```python
from build123d import *

# Parameters (mm, degrees)
SKETCH058_R     = 1.75
PAD036_DEPTH    = 5
SKETCH059_R     = 1.75
PAD037_DEPTH    = 0.6
SKETCH060_R     = 3
POCKET018_DEPTH = 3
SKETCH064_W     = 25
SKETCH064_H     = 15
POCKET020_DEPTH = 5
SKETCH065_W     = 32
SKETCH065_H     = 32
SKETCH065_W_2   = 25
SKETCH065_H_2   = 15
PAD040_DEPTH    = 3
POCKET021_DEPTH = 2
SKETCH067_W     = 32
SKETCH067_H     = 1.8
PAD041_DEPTH    = 2
SKETCH069_W     = 7.6
SKETCH069_H     = 1.2
PAD042_DEPTH    = 5
SKETCH070_R     = 1
POCKET022_DEPTH = 0.601
PAD043_DEPTH    = 10


with BuildPart() as part:
    # Sketch058 → Pad036 (new body)
    with BuildSketch(Plane.XY):
        Polygon((-42, 37.5), (12, 37.5), (12, 25.7), (42, 25.7), (42, -37.5), (-42, -37.5), align=None)
        with Locations((-15, 31.5)):
            Circle(SKETCH058_R, mode=Mode.SUBTRACT)
        with BuildLine():
            ThreePointArc((-18.5, 31.5), (-15, 28), (-11.5, 31.5))
            Line((-11.5, 31.5), (-11.5, 36.3))
            Line((-11.5, 36.3), (10.8, 36.3))
            Line((10.8, 36.3), (10.8, 24.5))
            Line((10.8, 24.5), (40.8, 24.5))
            Line((40.8, 24.5), (40.8, -36.3))
            Line((40.8, -36.3), (-40.8, -36.3))
            Line((-40.8, -36.3), (-40.8, 36.3))
            Line((-40.8, 36.3), (-18.5, 36.3))
            Line((-18.5, 31.5), (-18.5, 36.3))
        make_face(mode=Mode.SUBTRACT)
    extrude(amount=PAD036_DEPTH)

    # Sketch059 (on Face19 of Pad036) → Pad037 (join)
    with BuildSketch(Plane.XY.offset(5)):
        Polygon((-42, 37.5), (12, 37.5), (12, 25.7), (42, 25.7), (42, -37.5), (-42, -37.5), align=None)
        with Locations((-15, 31.5)):
            Circle(SKETCH059_R, mode=Mode.SUBTRACT)
    extrude(amount=PAD037_DEPTH)

    # Sketch060 (on Face1 of Pad037) → Pocket018 (cut)
    with BuildSketch(Plane.XY.offset(5.6)):
        with Locations((-15, 31.5)):
            Circle(SKETCH060_R)
    extrude(amount=-POCKET018_DEPTH, mode=Mode.SUBTRACT)

    # Sketch064 → Pocket020 (cut)
    with BuildSketch(Plane(origin=(0, 0, 5), x_dir=(1, 0, 0), z_dir=(0, 0, -1))):
        with Locations((-12.5, -7.5)):
            Rectangle(SKETCH064_W, SKETCH064_H)
    extrude(amount=-POCKET020_DEPTH, mode=Mode.SUBTRACT)

    # Sketch065 (on Face14 of Pocket020) → Pad040 (join)
    with BuildSketch(Plane(origin=(0, 0, 5), x_dir=(1, 0, 0), z_dir=(0, 0, -1))):
        with Locations((-12.5, -5)):
            Rectangle(SKETCH065_W, SKETCH065_H)
        with Locations((-12.5, -7.5)):
            Rectangle(SKETCH065_W_2, SKETCH065_H_2, mode=Mode.SUBTRACT)
    extrude(amount=PAD040_DEPTH)

    # Sketch066 (on Face24 of Pad040) → Pocket021 (cut)
    with BuildSketch(Plane(origin=(0, 0, 2), x_dir=(1, 0, 0), z_dir=(0, 0, -1))):
        Polygon((-26.75, -15.5), (-26.75, 5.5), (-21.75, 5.5), (-21.75, 9), (-3.25, 9), (-3.25, 5.5), (1.75, 5.5), (1.75, -15.5), (-3.25, -15.5), (-3.25, -19), (-21.75, -19), (-21.75, -15.5), align=None)
    extrude(amount=-POCKET021_DEPTH, mode=Mode.SUBTRACT)

    # Sketch067 (on Face40 of Pocket021) → Pad041 (join)
    with BuildSketch(Plane(origin=(0, 0, 2), x_dir=(1, 0, 0), z_dir=(0, 0, -1))):
        with Locations((-12.5, 10.1)):
            Rectangle(SKETCH067_W, SKETCH067_H)
        with Locations((-12.5, -20.1)):
            Rectangle(SKETCH067_W, SKETCH067_H)
    extrude(amount=PAD041_DEPTH)

    # Sketch069 (on Face13 of Pad041) → Pad042 (join)
    with BuildSketch(Plane(origin=(0, 0, 0), x_dir=(1, 0, 0), z_dir=(0, 0, -1))):
        with Locations((20.82, -25.1)):
            Rectangle(SKETCH069_W, SKETCH069_H)
    extrude(amount=PAD042_DEPTH)

    # Sketch070 (on Face40 of Pad042) → Pocket022 (cut, through all)
    with BuildSketch(Plane(origin=(0, 0, 5), x_dir=(1, 0, 0), z_dir=(0, 0, -1))):
        with Locations((24.892975, 0)):
            Circle(SKETCH070_R)
        with Locations((24.892975, -6)):
            Circle(SKETCH070_R)
        with Locations((24.892975, 6)):
            Circle(SKETCH070_R)
        with Locations((24.892975, 12)):
            Circle(SKETCH070_R)
    extrude(amount=-POCKET022_DEPTH, mode=Mode.SUBTRACT)

    # Sketch071 (on Face22 of Pocket022) → Pad043 (join)
    with BuildSketch(Plane(origin=(0, 0, 5), x_dir=(1, 0, 0), z_dir=(0, 0, -1))):
        with BuildLine():
            ThreePointArc((10.8, -32.3), (7.971573, -33.471573), (6.8, -36.3))
            Line((6.8, -36.3), (10.8, -36.3))
            Line((10.8, -36.3), (10.8, -32.3))
        make_face()
        with BuildLine():
            ThreePointArc((40.8, -20.5), (37.971573, -21.671573), (36.8, -24.5))
            Line((40.8, -24.5), (36.8, -24.5))
            Line((40.8, -20.5), (40.8, -24.5))
        make_face()
        with BuildLine():
            ThreePointArc((36.8, 36.3), (37.971573, 33.471573), (40.8, 32.3))
            Line((40.8, 36.3), (40.8, 32.3))
            Line((36.8, 36.3), (40.8, 36.3))
        make_face()
        with BuildLine():
            ThreePointArc((-40.8, 32.3), (-37.971573, 33.471573), (-36.8, 36.3))
            Line((-40.8, 36.3), (-36.8, 36.3))
            Line((-40.8, 32.3), (-40.8, 36.3))
        make_face()
        with BuildLine():
            ThreePointArc((-36.8, -36.3), (-37.971573, -33.471573), (-40.8, -32.3))
            Line((-40.8, -32.3), (-40.8, -36.3))
            Line((-36.8, -36.3), (-40.8, -36.3))
        make_face()
    extrude(amount=PAD043_DEPTH)


solid = part.part
```
Here's how the part is built. I have some questions about the finished solid (model axes, mm). A direction names the side the tool comes from. Coordinates: 2 decimals unless noted, no trailing zeros. Order: outer loops, then holes, each group sorted by start corner. A loop starts at its lowest first (then second) coordinate and runs counter-clockwise, first axis right, second up. Notation, with made-up numbers: (38.25, 42) - (55.25, 42) arc R12 ccw to (55.25, 54) - close; hole circle Ø2 at (54, 29.5). An arc over 180 degrees is marked (long way). One line per question, with ' | ' between items. Start each with the question number.
1. If we section it at D-D (x = -6.5): Write out the boundary of the cut face in (y, z).
2. Which directions (+Z, -Z, +X, -X, +Y, -Y) give clear straight access to the entire face, cutting with the end or side of a thin tool? Please do faces 4 (the flat face through (39, 24.5, -2)), 5 (the flat face through (-18.5, 34, 2)), 6 (the flat face through (27, 25.7, 1)).
3. If we section it at C-C (z = -2): Write out the boundary of the cut face in (x, y), and give its area (3 significant figures).
4. Please list where these lines run through material, in increasing order: line 1 along X through (y, z) = (-2, 2.25); line 2 along X through (y, z) = (6, 5.45); line 3 along Y through (x, z) = (-15, 3.9). Write a range as [from, to].
5. If we section it at A-A (y = -12): Write out the boundary of the cut face in (x, z), and give its area (3 significant figures).
6. If we mould it in two halves opening along Y, with no side actions, what happens to faces 1 (the flat face through (-40.8, 34, -2)), 2 (the flat face through (10.8, 28, 2)), 3 (the flat face through (-39, -36.3, -2))? For each: released by +Y, released by -Y, zero draft, split by the parting line, or undercut.
7. If we section it at B-B (x = -15): Give the number of separate pieces and of enclosed holes in the cut face, and give its area (3 significant figures).
8. I'm going to push flat-ended pins straight in: pin 1 Ø2 at (y, z) = (-34, -3.5) entering from +X; pin 2 Ø1.2 at (x, z) = (39.5, -2) entering from -Y; pin 3 Ø2 at (y, z) = (35, -3) entering from -X. Where does each tip first touch, or does it pass through?
Model answer:
1) outline: (-37.5, 0) - (-36.3, 0) - (-36.3, 5) - (-11, 5) - (-11, 0) - (-9.2, 0) - (-9.2, 2) - (-9, 2) - (-9, 4) - (0, 4) - (0, 5.6) - (-37.5, 5.6) - close; (15, 4) - (19, 4) - (19, 2) - (19.2, 2) - (19.2, 0) - (21, 0) - (21, 5) - (36.3, 5) - (36.3, 0) - (37.5, 0) - (37.5, 5.6) - (15, 5.6) - close
2) face 4: -Z, +X, +Y | face 5: -Z | face 6: +Z, -Z, +X, +Y
3) outline: (-40.8, -36.3) - (-36.8, -36.3) arc R4 ccw to (-40.8, -32.3) - close; (-40.8, 32.3) arc R4 ccw to (-36.8, 36.3) - (-40.8, 36.3) - close; (6.8, 36.3) arc R4 ccw to (10.8, 32.3) - (10.8, 36.3) - close; (17.02, 24.5) - (24.62, 24.5) - (24.62, 25.7) - (17.02, 25.7) - close; (36.8, -36.3) - (40.8, -36.3) - (40.8, -32.3) arc R4 ccw to start; (36.8, 24.5) arc R4 ccw to (40.8, 20.5) - (40.8, 24.5) - close | area: 72.0 mm²
4) line 1: x = [-42, -40.8], [-28.5, -26.75], [1.75, 3.5], [40.8, 42] | line 2: x = [-42, -25], [0, 23.89], [25.89, 42] | line 3: y = [-37.5, -36.3], [-11, -9], [19, 21], [28, 28.5], [34.5, 37.5]
5) outline: (-42, 0) - (-40.8, 0) - (-40.8, 5) - (23.89, 5) - (23.89, 5.6) - (-42, 5.6) - close; (25.89, 5) - (40.8, 5) - (40.8, 0) - (42, 0) - (42, 5.6) - (25.89, 5.6) - close | area: 61.2 mm²
6) face 1: zero draft | face 2: undercut | face 3: released by -Y
7) separate pieces: 3 | enclosed holes: 0 | area: 94.6 mm²
8) pin 1: stops at x = 40.8 | pin 2: stops at y = -36.3 | pin 3: stops at x = -40.8
